Verification items for the finished model (mm, model axes). A direction names the side the tool comes from. Round coordinates to 2 decimals unless told otherwise and drop trailing zeros. Order: outer loops, then holes, each group sorted by start corner. A loop starts at its lowest first (then second) coordinate and runs counter-clockwise, first axis right, second up. Notation, with made-up numbers: (-18, 20.25) -> (21, 20.25) arc R30 ccw to (21, 45.25) -> close; hole circle Ø10 at (-8, 63). An arc over 180 degrees is marked (long way). Put each result on its own line as item: value.
```python
from build123d import *

# Parameters (mm, degrees)
SKETCH1_R           = 4.7625
BASE_EXTRUDE_DEPTH  = 50.8
SKETCH2_R           = 4.7625
BOSS_EXTRUDE1_DEPTH = 5.08
BOSS_EXTRUDE1_TAPER = -45
SKETCH3_W           = 1.754126852
SKETCH3_H           = 4.225851054
CUT_EXTRUDE1_DEPTH  = 3.175
CIRPATTERN1_COUNT   = 4
SKETCH4_R           = 9.8425
BOSS_EXTRUDE2_DEPTH = 0.762
CHAMFER1_SIZE       = 2.54


with BuildPart() as part:
    # Sketch1 → Base-Extrude (new body)
    with BuildSketch(Plane.XY):
        Circle(SKETCH1_R)
    extrude(amount=BASE_EXTRUDE_DEPTH)

    # Sketch2 → Boss-Extrude1 (add)
    with BuildSketch(Plane(origin=(0, 0, 0), x_dir=(-1, 0, 0), z_dir=(0, 0, -1))):
        Circle(SKETCH2_R)
    extrude(amount=BOSS_EXTRUDE1_DEPTH, taper=BOSS_EXTRUDE1_TAPER)

    # Sketch3 → Cut-Extrude1 (cut)
    with BuildSketch(Plane(origin=(0, 0, -5.08), x_dir=(-1, 0, 0), z_dir=(0, 0, -1))):
        with Locations((0, 2.112925527)):
            Rectangle(SKETCH3_W, SKETCH3_H)
    cut_extrude1 = extrude(amount=-CUT_EXTRUDE1_DEPTH, mode=Mode.SUBTRACT)

    # CirPattern1: Cut-Extrude1 ×4 about axis
    cirpattern1_axis = Axis((0, 0, 0), (0, 0, -1))
    for i in range(1, CIRPATTERN1_COUNT):
        add(cut_extrude1.rotate(cirpattern1_axis, i * 360 / CIRPATTERN1_COUNT), mode=Mode.SUBTRACT)

    # Sketch4 → Boss-Extrude2 (add)
    with BuildSketch(Plane(origin=(0, 0, -5.08), x_dir=(-1, 0, 0), z_dir=(0, 0, -1))):
        Circle(SKETCH4_R)
        Polygon((-0.877063426, 0.877063426), (-4.225851054, 0.877063426), (-4.225851054, -0.877063426), (-0.877063426, -0.877063426), (-0.877063426, -4.225851054), (0.877063426, -4.225851054), (0.877063426, -0.877063426), (4.225851054, -0.877063426), (4.225851054, 0.877063426), (0.877063426, 0.877063426), (0.877063426, 4.225851054), (-0.877063426, 4.225851054), align=None, mode=Mode.SUBTRACT)
    extrude(amount=BOSS_EXTRUDE2_DEPTH)

    # Chamfer1
    chamfer1_edges = [part.edges().sort_by_distance(p)[0] for p in [
        (-4.7625, 0, 50.8),
    ]]
    chamfer(chamfer1_edges, length=CHAMFER1_SIZE)


solid = part.part
```
Item 1: Depth check by flat-ended pin: pin 1 Ø0.5 at (y, z) = (0, -4.5) entering from +X; pin 2 Ø4 at (y, z) = (-0.5, 8) entering from -X; pin 3 Ø1.9 at (x, z) = (0.5, -3.5) entering from -Y. Enter the tip coordinate at first touch or a pass-through.
Geometry check:
pin 1: x = 9.51
pin 2: x = -4.76
pin 3: y = -9.2
Item 2: Material ranges on line 1 along Z through (x, y) = (0.5, -2) (3 decimals); line 2 along X through (y, z) = (3.5, 41.5); line 3 along Y through (x, z) = (0.75, -1.5), recorded low to high.
Geometry check:
line 1: -1.905 to 50.8
line 2: -3.23 to 3.23
line 3: -6.22 to 6.22
Item 3: Release check for a two-part mould opening along X. For faces 4 (the face through (7.8, -6, -5.5)), 5 (the face through (0, 0, 50.8)), 6 (the face through (-0.877, -3, -4)) record: pulls with the +X half, pulls with the -X half, needs draft (parallel to the pull), parting line crosses it, or undercut.
Geometry check:
face 4: parting line crosses it
face 5: needs draft
face 6: undercut
Item 4: Sectioned sample at A-A, the plane x = 0. Record the boundary of the cut face in (y, z) (1 decimal), then the cut area to 3 significant figures.
Geometry check:
outline: (-9.8, -5.8) -> (-4.2, -5.8) -> (-4.2, -1.9) -> (4.2, -1.9) -> (4.2, -5.8) -> (9.8, -5.8) -> (9.8, -5.1) -> (4.8, 0) -> (4.8, 48.3) -> (2.2, 50.8) -> (-2.2, 50.8) -> (-4.8, 48.3) -> (-4.8, 0) -> (-9.8, -5.1) -> close
area: 533 mm2
Item 5: Sectioned sample at B-B, the plane z = 18. Record the boundary of the cut face in (x, y) (1 decimal), then the cut area to 3 significant figures.
Geometry check:
outline: circle Ø9.5 at (0, 0)
area: 71.3 mm2
Item 6: Tool access check on faces 1 (the face through (-3.78, -2.9, 23.79)), 2 (the face through (-2, -2, -5.842)), 3 (the face through (0, 4.226, -4)). Record the directions out of +Z, -Z, +X, -X, +Y, -Y that give a thin tool (end or side, any length) a straight path to the whole face; none if there is none.
Geometry check:
face 1: +Z
face 2: -Z, +X, -X, +Y, -Y
face 3: -Z
